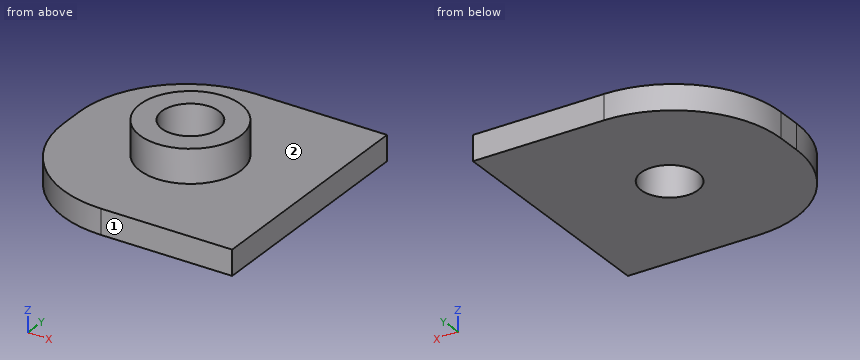
```python
from build123d import *

# Parameters (mm, degrees)
SKETCH1_W           = 18.034
SKETCH1_H           = 18.034
SKETCH1_R           = 2.15265
BOSS_EXTRUDE1_DEPTH = 1.905
SKETCH2_R           = 3.81
SKETCH2_R_2         = 2.15265
BOSS_EXTRUDE2_DEPTH = 2.54
CUT_EXTRUDE1_DEPTH  = 14.504466039


with BuildPart() as part:
    # Sketch1 → Boss-Extrude1 (new body)
    with BuildSketch(Plane.XY):
        Rectangle(SKETCH1_W, SKETCH1_H)
        with Locations(Location((0, 0, 0), (0, 0, 180))):
            Circle(SKETCH1_R, mode=Mode.SUBTRACT)
    extrude(amount=BOSS_EXTRUDE1_DEPTH)

    # Sketch2 → Boss-Extrude2 (add)
    with BuildSketch(Plane.XY.offset(1.905)):
        with Locations(Location((0, 0, 0), (0, 0, 180))):
            Circle(SKETCH2_R)
        with Locations(Location((0, 0, 0), (0, 0, 180))):
            Circle(SKETCH2_R_2, mode=Mode.SUBTRACT)
    extrude(amount=BOSS_EXTRUDE2_DEPTH)

    # Sketch3 → Cut-Extrude1 (cut, through all)
    with BuildSketch(Plane(origin=(0, 0, 0), x_dir=(-1, 0, 0), z_dir=(0, 0, -1))):
        with BuildLine():
            Line((9.017, 0.904485111), (9.017, 9.017))
            Line((9.017, 9.017), (0.904485111, 9.017))
            ThreePointArc((0.904485111, 9.017), (6.640899402, 6.640899402), (9.017, 0.904485111))
        make_face()
        with BuildLine():
            Line((9.017, -9.017), (0.904485111, -9.017))
            ThreePointArc((0.904485111, -9.017), (6.640899402, -6.640899402), (9.017, -0.904485111))
            Line((9.017, -0.904485111), (9.017, -9.017))
        make_face()
    extrude(amount=-CUT_EXTRUDE1_DEPTH, mode=Mode.SUBTRACT)


solid = part.part
```
Build history of the part. All positions in model axes, mm. Face numbers are marked on the shaded views. A direction names the side the tool comes from. Give positions to 0.01 mm unless a question says otherwise; leave off trailing zeros. Loops run counter-clockwise (first coordinate to the right, second up) from the corner with the lowest first, then second, coordinate; pieces in that order, holes last.
1) Band-saw the part on D-D on x = 2.75. List the corners of the cut face in (y, z) (3 decimals).
Values follow:
outline: (-9.017, 0) - (9.017, 0) - (9.017, 1.905) - (2.637, 1.905) - (2.637, 4.445) - (-2.637, 4.445) - (-2.637, 1.905) - (-9.017, 1.905) - close
2) Drop a flat-ended pin along its axis: P1, Ø1.5, axis at y = -7, z = 2.5, coming from the -X side. Give the stop position or say it passes through.
Values follow:
P1: stops at x = -6.74
3) Band-saw the part on A-A on x = 0. List the corners of the cut face in (y, z) (3 decimals).
Values follow:
outline: (-9.017, 0) - (-2.153, 0) - (-2.153, 4.445) - (-3.81, 4.445) - (-3.81, 1.905) - (-9.017, 1.905) - close; (2.153, 0) - (9.017, 0) - (9.017, 1.905) - (3.81, 1.905) - (3.81, 4.445) - (2.153, 4.445) - close
4) Probe line 1 along Y through (x, z) = (0, 3); line 2 along Y through (x, z) = (0, 1.7); line 3 along Z through (x, y) = (2.5, 8.25) (3 decimals). List the from-to ranges inside material, lowest first.
Values follow:
line 1: y = -3.81 to -2.15, 2.15 to 3.81
line 2: y = -9.02 to -2.15, 2.15 to 9.02
line 3: z = 0 to 1.905
5) Band-saw the part on C-C on z = 0.8. List the corners of the cut face in (x, y), then the cut area to 3 significant figures.
Values follow:
outline: (-9.02, -0.9) arc R8.11 ccw to (-0.9, -9.02) - (9.02, -9.02) - (9.02, 9.02) - (-0.9, 9.02) arc R8.11 ccw to (-9.02, 0.9) - close; hole circle Ø4.31 at (0, 0)
area: 282 mm2
6) 3-axis set-ups, long thin cutter, end or side, ignore diameter. For the marked faces 1 and 2: which of +Z, -Z, +X, -X, +Y, -Y reach the whole face in a straight line?
Values follow:
face 1: +Z, -Z, +X, -X, -Y
face 2: +Z
